Input: part model. Units: mm. Frame: model coordinates. Face numbers are marked on the shaded views. A direction names the side the tool comes from. Coordinates: 2 decimals unless noted, no trailing zeros. Write each loop counter-clockwise with the first axis right and the second up, starting at its lowest first coordinate (ties: lowest second). Pieces come first, ordered by that corner, then holes.
1) Pin query (flat end, axial travel): pin 1 Ø1 at (x, z) = (13, -19) entering from +Y; pin 2 Ø10 at (x, y) = (25, 14.5) entering from +Z; pin 3 Ø5 at (y, z) = (17.5, 1.5) entering from -X. Return the tip coordinate at first contact, or that it passes through.
2) Set-up query: the marked faces 4 and 5. Return all of +Z, -Z, +X, -X, +Y, -Y with unobstructed straight access to the full face (end or side cutting, diameter ignored); none if empty.
3) Draft query along X for the marked faces 1, 2 and 3. Return one class per face: pulls with the +X half, pulls with the -X half, needs draft (parallel to the pull), parting line crosses it, or undercut.
4) Section query B-B (z = 11). State how many separate pieces and enclosed holes the cut face has, then the cut area to 3 significant figures.
5) Section query A-A (x = 10). Output: boundary loops of the cut face in (y, z), then the cut area to 3 significant figures.
6) Line query: L1, parallel to Z at x = -1.5, y = 15.25; L2, parallel to Y at x = -61.5, z = 0; L3, parallel to X at y = 5.5, z = 15. Output: solid intervals per line, ascending.
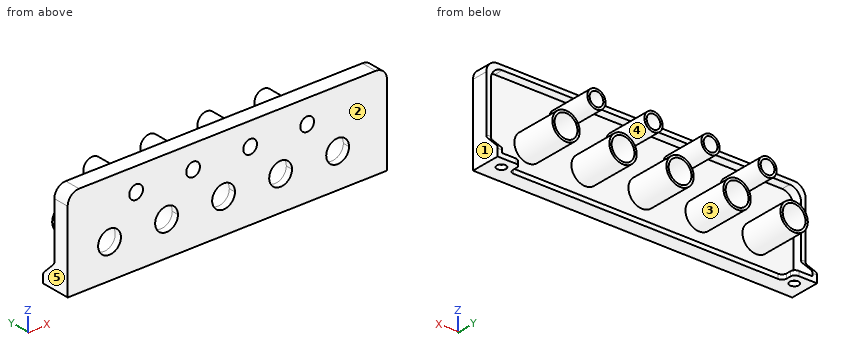
from build123d import *

# Parameters (mm, degrees)
ESQUISSE1_W                      = 140
ESQUISSE1_H                      = 40
BOSS_EXTRU_1_DEPTH               = 3
ESQUISSE2_R                      = 6
ESQUISSE2_R_2                    = 5
BOSS_EXTRU_2_DEPTH               = 20
ESQUISSE7_R                      = 5
ENL_V_MAT_EXTRU_3_DEPTH          = 76.498344353
R_P_TITION_LIN_AIRE3_OUTLINE_R   = 5
R_P_TITION_LIN_AIRE3_DEPTH       = 3
R_P_TITION_START                 = 3
R_P_TITION_LIN_AIRE3_2_OUTLINE_R = 6
R_P_TITION_LIN_AIRE3_2_DEPTH     = 20
ESQUISSE8_R                      = 5
ENL_V_MAT_EXTRU_4_DEPTH          = 77.347887987
R_P_TITION_LIN_AIRE4_COUNT       = 4
R_P_TITION_LIN_AIRE4_PITCH       = 25
ESQUISSE9_R                      = 4
BOSS_EXTRU_4_DEPTH               = 20
ESQUISSE12_R                     = 3
ENL_V_MAT_EXTRU_6_DEPTH          = 77.347887987
R_P_TITION_LIN_AIRE5_COUNT       = 4
R_P_TITION_LIN_AIRE5_PITCH       = 25
BOSS_EXTRU_5_DEPTH               = 10
CHANFREIN1_SIZE                  = 6
ESQUISSE15_R                     = 2
ENL_V_MAT_EXTRU_7_DEPTH          = 83.903558428
ESQUISSE18_W                     = 60
ESQUISSE18_H                     = 2
BOSS_EXTRU_6_DEPTH               = 4
CONG_2_R                         = 5
CONG_3_R                         = 2
SYM_TRIE1_OUTLINE_W              = 4
SYM_TRIE1_OUTLINE_H              = 2
SYM_TRIE1_DEPTH                  = 62.191181732
SYM_TRIE1_START                  = 68
SYM_TRIE1_2_DEPTH                = 2
SYM_TRIE1_START_2                = 66.191181932
SYM_TRIE1_3_OUTLINE_W            = 10
SYM_TRIE1_3_OUTLINE_H            = 2
SYM_TRIE1_3_OUTLINE_W_2          = 4
SYM_TRIE1_3_DEPTH                = 1.808818068
SYM_TRIE1_START_3                = 62
SYM_TRIE1_4_OUTLINE_W            = 4
SYM_TRIE1_4_OUTLINE_H            = 2
SYM_TRIE1_4_DEPTH                = 6
SYM_TRIE1_5_OUTLINE_W            = 6
SYM_TRIE1_5_OUTLINE_H            = 2
SYM_TRIE1_5_DEPTH                = 0.191181732
SYM_TRIE1_START_4                = -20
SYM_TRIE1_6_DEPTH                = 2
SYM_TRIE1_START_5                = 2
SYM_TRIE1_7_DEPTH                = 5
CONG_4_R                         = 5


with BuildPart() as part:
    # Esquisse1 → Boss.-Extru.1 (new body)
    with BuildSketch(Plane(origin=(0, 0, 0), x_dir=(1, 0, 0), z_dir=(0, 1, 0))):
        Rectangle(ESQUISSE1_W, ESQUISSE1_H)
    extrude(amount=BOSS_EXTRU_1_DEPTH)

    # Esquisse2 → Boss.-Extru.2 (add)
    with BuildSketch(Plane(origin=(0, 3, 0), x_dir=(1, 0, 0), z_dir=(0, 1, 0))):
        with Locations(Location((-51.645903367, 5, 0), (0, 0, 270))):
            Circle(ESQUISSE2_R)
        with Locations(Location((-51.645903367, 5, 0), (0, 0, 270))):
            Circle(ESQUISSE2_R_2, mode=Mode.SUBTRACT)
    extrude(amount=BOSS_EXTRU_2_DEPTH)

    # Esquisse7 → Enlèv. mat.-Extru.3 (cut, through all)
    with BuildSketch(Plane(origin=(0, 3, 0), x_dir=(1, 0, 0), z_dir=(0, 1, 0))):
        with Locations(Location((-51.645903367, 5, 0), (0, 0, 270))):
            Circle(ESQUISSE7_R)
    extrude(amount=-ENL_V_MAT_EXTRU_3_DEPTH, mode=Mode.SUBTRACT)

    # Répétition linéaire3: read off the stored shape, not the designer's step
    # Répétition linéaire3 outline → Répétition linéaire3 (cut)
    with BuildSketch(Plane(origin=(0, 0, 0), x_dir=(1, 0, 0), z_dir=(0, 1, 0))):
        with Locations((-26.645903367, 5)):
            Circle(R_P_TITION_LIN_AIRE3_OUTLINE_R)
        with Locations((48.354096633, 5)):
            Circle(R_P_TITION_LIN_AIRE3_OUTLINE_R)
        with Locations((23.354096633, 5)):
            Circle(R_P_TITION_LIN_AIRE3_OUTLINE_R)
        with Locations((-1.645903367, 5)):
            Circle(R_P_TITION_LIN_AIRE3_OUTLINE_R)
    extrude(amount=R_P_TITION_LIN_AIRE3_DEPTH, mode=Mode.SUBTRACT)

    # R_p_tition lin_aire3 2 outline → R_p_tition lin_aire3 2 (add)
    with BuildSketch(Plane(origin=(0, 0, 0), x_dir=(1, 0, 0), z_dir=(0, 1, 0)).offset(R_P_TITION_START)):
        with Locations((48.354096633, 5)):
            Circle(R_P_TITION_LIN_AIRE3_2_OUTLINE_R)
        with Locations((23.354096633, 5)):
            Circle(R_P_TITION_LIN_AIRE3_2_OUTLINE_R)
        with Locations((-1.645903367, 5)):
            Circle(R_P_TITION_LIN_AIRE3_2_OUTLINE_R)
        with Locations((-26.645903367, 5)):
            Circle(R_P_TITION_LIN_AIRE3_2_OUTLINE_R)
    extrude(amount=R_P_TITION_LIN_AIRE3_2_DEPTH)

    # Esquisse8 → Enlèv. mat.-Extru.4 (cut, through all)
    with BuildSketch(Plane(origin=(0, 23, 0), x_dir=(1, 0, 0), z_dir=(0, 1, 0))):
        with Locations(Location((-26.645903367, 5, 0), (0, 0, 270))):
            Circle(ESQUISSE8_R)
    enl_v_mat_extru_4 = extrude(amount=-ENL_V_MAT_EXTRU_4_DEPTH, mode=Mode.SUBTRACT)

    # Répétition linéaire4: Enlèv. mat.-Extru.4 ×4
    with Locations(*[(i * R_P_TITION_LIN_AIRE4_PITCH, 0, 0) for i in range(1, R_P_TITION_LIN_AIRE4_COUNT)]):
        add(enl_v_mat_extru_4, mode=Mode.SUBTRACT)

    # Esquisse9 → Boss.-Extru.4 (add)
    with BuildSketch(Plane(origin=(0, 3, 0), x_dir=(1, 0, 0), z_dir=(0, 1, 0))):
        with Locations(Location((-40, -10.001459341, 0), (0, 0, 270))):
            Circle(ESQUISSE9_R)
    boss_extru_4 = extrude(amount=BOSS_EXTRU_4_DEPTH)

    # Esquisse12 → Enlèv. mat.-Extru.6 (cut, through all)
    with BuildSketch(Plane(origin=(0, 23, 0), x_dir=(1, 0, 0), z_dir=(0, 1, 0))):
        with Locations(Location((-40, -10.001459341, 0), (0, 0, 270))):
            Circle(ESQUISSE12_R)
    enl_v_mat_extru_6 = extrude(amount=-ENL_V_MAT_EXTRU_6_DEPTH, mode=Mode.SUBTRACT)

    # Répétition linéaire5: Boss.-Extru.4, Enlèv. mat.-Extru.6 ×4
    with Locations(*[(i * R_P_TITION_LIN_AIRE5_PITCH, 0, 0) for i in range(1, R_P_TITION_LIN_AIRE5_COUNT)]):
        add(boss_extru_4)
        add(enl_v_mat_extru_6, mode=Mode.SUBTRACT)

    # Esquisse13 → Boss.-Extru.5 (add)
    with BuildSketch(Plane(origin=(0, 3, 0), x_dir=(1, 0, 0), z_dir=(0, 1, 0))):
        Polygon((-70, 20), (-60, 20), (-60, 18), (-68, 18), (-68, 10), (-70, 10), align=None)
    extrude(amount=BOSS_EXTRU_5_DEPTH)

    # Chanfrein1
    chanfrein1_edges = [part.edges().sort_by_distance(p)[0] for p in [
        (-69, 13, -10),
    ]]
    chamfer(chanfrein1_edges, length=CHANFREIN1_SIZE)

    # Esquisse15 → Enlèv. mat.-Extru.7 (cut, through all)
    with BuildSketch(Plane.XY.offset(-18)):
        with Locations((-64.191181832, 8)):
            Circle(ESQUISSE15_R)
    extrude(amount=-ENL_V_MAT_EXTRU_7_DEPTH, mode=Mode.SUBTRACT)

    # Esquisse18 → Boss.-Extru.6 (add)
    with BuildSketch(Plane(origin=(0, 3, 0), x_dir=(1, 0, 0), z_dir=(0, 1, 0))):
        Polygon((-68, 10), (-68, -18), (0, -18), (0, -20), (-70, -20), (-70, 10), align=None)
        with Locations((-30, 19)):
            Rectangle(ESQUISSE18_W, ESQUISSE18_H)
    extrude(amount=BOSS_EXTRU_6_DEPTH)

    # Congé2
    cong_2_edges = [part.edges().sort_by_distance(p)[0] for p in [
        (-68, 5, 18),
        (-70, 3.5, 20),
    ]]
    fillet(cong_2_edges, radius=CONG_2_R)

    # Congé3
    cong_3_edges = [part.edges().sort_by_distance(p)[0] for p in [
        (-60, 13, -19),
        (-69, 13, -16),
        (-69, 7, -10),
        (-60, 7, -19),
    ]]
    fillet(cong_3_edges, radius=CONG_3_R)

    # Symétrie1: read off the stored shape, not the designer's step
    # Symétrie1 outline → Symétrie1 (add)
    with BuildSketch(Plane.YZ):
        with Locations((5, -19)):
            Rectangle(SYM_TRIE1_OUTLINE_W, SYM_TRIE1_OUTLINE_H)
        with Locations((5, 19)):
            Rectangle(SYM_TRIE1_OUTLINE_W, SYM_TRIE1_OUTLINE_H)
    extrude(amount=SYM_TRIE1_DEPTH)

    # Sym_trie1 2 outline → Sym_trie1 2 (add)
    with BuildSketch(Plane.YZ.offset(SYM_TRIE1_START)):
        with BuildLine():
            Line((13, -20), (13, -16.828427125))
            ThreePointArc((13, -16.828427125), (12.847759065, -16.06306026), (12.414213562, -15.414213562))
            Line((12.414213562, -15.414213562), (7.585786438, -10.585786438))
            ThreePointArc((7.585786438, -10.585786438), (7.152240935, -9.93693974), (7, -9.171572875))
            Line((7, -9.171572875), (7, 20))
            Line((7, 20), (3, 20))
            Line((3, 20), (3, -20))
            Line((3, -20), (13, -20))
        make_face()
    extrude(amount=SYM_TRIE1_2_DEPTH)

    # Sym_trie1 3 outline → Sym_trie1 3 (add)
    with BuildSketch(Plane.YZ.offset(SYM_TRIE1_START_2)):
        with Locations((8, -19)):
            Rectangle(SYM_TRIE1_3_OUTLINE_W, SYM_TRIE1_3_OUTLINE_H)
        with Locations((5, 19)):
            Rectangle(SYM_TRIE1_3_OUTLINE_W_2, SYM_TRIE1_3_OUTLINE_H)
    extrude(amount=SYM_TRIE1_3_DEPTH)

    # Sym_trie1 4 outline → Sym_trie1 4 (add)
    with BuildSketch(Plane.YZ.offset(SYM_TRIE1_START_3)):
        with Locations((5, 19)):
            Rectangle(SYM_TRIE1_4_OUTLINE_W, SYM_TRIE1_4_OUTLINE_H)
    extrude(amount=SYM_TRIE1_4_DEPTH)

    # Sym_trie1 5 outline → Sym_trie1 5 (add)
    with BuildSketch(Plane.YZ.offset(SYM_TRIE1_START_3)):
        with Locations((10, -19)):
            Rectangle(SYM_TRIE1_5_OUTLINE_W, SYM_TRIE1_5_OUTLINE_H)
    extrude(amount=SYM_TRIE1_5_DEPTH)

    # Sym_trie1 6 outline → Sym_trie1 6 (add)
    with BuildSketch(Plane.XY.offset(SYM_TRIE1_START_4)):
        with BuildLine():
            ThreePointArc((62, 13), (60.585786438, 12.414213562), (60, 11))
            Line((60, 11), (60, 9))
            ThreePointArc((60, 9), (59.414213562, 7.585786438), (58, 7))
            Line((58, 7), (62, 7))
            Line((62, 7), (62, 13))
        make_face()
        with BuildLine():
            Line((66.191181932, 13), (62.191181732, 13))
            Line((62.191181732, 13), (62.191181832, 8))
            ThreePointArc((62.191181832, 8), (64.191181832, 10), (66.191181832, 8))
            Line((66.191181832, 8), (66.191181932, 13))
        make_face()
        with BuildLine():
            Line((62.191181832, 8), (62.191181732, 3))
            Line((62.191181732, 3), (66.191181932, 3))
            Line((66.191181932, 3), (66.191181832, 8))
            ThreePointArc((66.191181832, 8), (64.191181832, 6), (62.191181832, 8))
        make_face()
    extrude(amount=SYM_TRIE1_6_DEPTH)

    # Sym_trie1 7 outline → Sym_trie1 7 (add)
    with BuildSketch(Plane(origin=(0, 0, 0), x_dir=(1, 0, 0), z_dir=(0, 1, 0)).offset(SYM_TRIE1_START_5)):
        with BuildLine():
            Line((68, -18), (68, -13))
            ThreePointArc((68, -13), (66.535533906, -16.535533906), (63, -18))
            Line((63, -18), (68, -18))
        make_face()
    extrude(amount=SYM_TRIE1_7_DEPTH)

    # Congé4
    cong_4_edges = [part.edges().sort_by_distance(p)[0] for p in [
        (70, 3.5, 20),
    ]]
    fillet(cong_4_edges, radius=CONG_4_R)


solid = part.part
Answer:
1. pin 1: stops at y = 7
1. pin 2: stops at z = 1
1. pin 3: stops at x = -56.12
2. face 4: +Y
2. face 5: +Z, -Z, -X, +Y, -Y
3. face 1: pulls with the +X half
3. face 2: needs draft
3. face 3: undercut
4. separate pieces: 5
4. enclosed holes: 0
4. area: 535 mm2
5. outline: (0, -20) - (7, -20) - (7, -18) - (3, -18) - (3, 6) - (23, 6) - (23, 7) - (0, 7) - close; (0, 13) - (23, 13) - (23, 14) - (3, 14) - (3, 18) - (7, 18) - (7, 20) - (0, 20) - close
5. area: 158 mm2
6. L1: z = -11 to -10, 0 to 1
6. L2: y = 0 to 3
6. L3: x = -70 to -67.58, 67.58 to 70
